Input: part model. Units: mm. Frame: model coordinates. Coordinates: 2 decimals unless noted, no trailing zeros. Order: outer loops, then holes, each group sorted by start corner. A loop starts at its lowest first (then second) coordinate and runs counter-clockwise, first axis right, second up.
from build123d import *

# Parameters (mm, degrees)
SKETCH2_W           = 73
SKETCH2_H           = 73
SKETCH2_R           = 4
BOSS_EXTRUDE1_DEPTH = 1.5
SKETCH3_R           = 1.5
CUT_EXTRUDE1_DEPTH  = 2.5
SKETCH4_R           = 1.5
CUT_EXTRUDE2_DEPTH  = 2.5
FILLET1_R           = 10


with BuildPart() as part:
    # Sketch2 → Boss-Extrude1 (new body)
    with BuildSketch(Plane(origin=(0, 0, 0), x_dir=(1, 0, 0), z_dir=(0, 1, 0))):
        Rectangle(SKETCH2_W, SKETCH2_H)
        Circle(SKETCH2_R, mode=Mode.SUBTRACT)
    extrude(amount=BOSS_EXTRUDE1_DEPTH)

    # Sketch3 → Cut-Extrude1 (cut, through all)
    with BuildSketch(Plane(origin=(0, 1.5, 0), x_dir=(1, 0, 0), z_dir=(0, 1, 0))):
        with Locations((-15.5, 15.5)):
            Circle(SKETCH3_R)
        with Locations((15.5, 15.5)):
            Circle(SKETCH3_R)
        with Locations((15.5, -15.5)):
            Circle(SKETCH3_R)
        with Locations((-15.5, -15.5)):
            Circle(SKETCH3_R)
    extrude(amount=-CUT_EXTRUDE1_DEPTH, mode=Mode.SUBTRACT)

    # Sketch4 → Cut-Extrude2 (cut, through all)
    with BuildSketch(Plane(origin=(0, 1.5, 0), x_dir=(1, 0, 0), z_dir=(0, 1, 0))):
        with Locations((-25, 25)):
            Circle(SKETCH4_R)
        with Locations((25, 25)):
            Circle(SKETCH4_R)
        with Locations((25, -25)):
            Circle(SKETCH4_R)
        with Locations((-25, -25)):
            Circle(SKETCH4_R)
    extrude(amount=-CUT_EXTRUDE2_DEPTH, mode=Mode.SUBTRACT)

    # Fillet1
    fillet1_edges = [part.edges().sort_by_distance(p)[0] for p in [
        (36.5, 0.75, 36.5),
        (-36.5, 0.75, 36.5),
        (-36.5, 0.75, -36.5),
        (36.5, 0.75, -36.5),
    ]]
    fillet(fillet1_edges, radius=FILLET1_R)


solid = part.part
Item 1: Cut plane C-C on x = 0. Return loops of the section in (y, z).
Response values:
outline: (0, -36.5) - (1.5, -36.5) - (1.5, -4) - (0, -4) - close; (0, 4) - (1.5, 4) - (1.5, 36.5) - (0, 36.5) - close
Item 2: Cut plane D-D on x = -25. Return loops of the section in (y, z), then the cut area to 4 significant figures.
Response values:
outline: (0, -36.5) - (1.5, -36.5) - (1.5, -26.5) - (0, -26.5) - close; (0, -23.5) - (1.5, -23.5) - (1.5, 23.5) - (0, 23.5) - close; (0, 26.5) - (1.5, 26.5) - (1.5, 36.5) - (0, 36.5) - close
area: 100.5 mm2
Item 3: Cut plane B-B on z = 25. Return loops of the section in (x, y), then the cut area to 4 significant figures.
Response values:
outline: (-36.5, 0) - (-26.5, 0) - (-26.5, 1.5) - (-36.5, 1.5) - close; (-23.5, 0) - (23.5, 0) - (23.5, 1.5) - (-23.5, 1.5) - close; (26.5, 0) - (36.5, 0) - (36.5, 1.5) - (26.5, 1.5) - close
area: 100.5 mm2
Item 4: Ray query, probe 1 along X at (y, z) = (0.9, 25); probe 2 along X at (y, z) = (0.9, 15.5). Return the intervals inside material, ascending.
Response values:
probe 1: x = -36.5 to -26.5, -23.5 to 23.5, 26.5 to 36.5
probe 2: x = -36.5 to -17, -14 to 14, 17 to 36.5
Item 5: Cut plane A-A on y = 0.9. Count the separate pieces of the cut face and the enclosed holes in it, then the cut area to 3 significant figures.
Response values:
separate pieces: 1
enclosed holes: 9
area: 5,140 mm2
Item 6: Draft query along X for faces 1 (the face through (8, 0, -1)), 2 (the face through (-17, 0.76, -15.57)), 3 (the face through (-33.65, 0.76, 33.49)), 4 (the face through (33.49, 0.76, -33.65)). Return one class per face: pulls with the +X half, pulls with the -X half, needs draft (parallel to the pull), parting line crosses it, or undercut.
Response values:
face 1: needs draft
face 2: undercut
face 3: pulls with the -X half
face 4: pulls with the +X half
